Source: CAD feature listing. Evaluate the final solid. Frame: model axes, mm. Round coordinates to 2 decimals unless told otherwise and drop trailing zeros. Order: outer loops, then holes, each group sorted by start corner. A loop starts at its lowest first (then second) coordinate and runs counter-clockwise, first axis right, second up. Notation, with made-up numbers: (-37.5, 63.5) -> (5.5, 63.5) arc R26 cw to (5.5, 88.5) -> close; hole circle Ø2 at (-39.75, 89). An arc over 180 degrees is marked (long way). Write item = value, one per line. Start each with the question number.
(1) Draft query along Y for faces 1 (the face through (0, 34.29, 6)), 2 (the face through (31.75, -17, 6)), 3 (the face through (1.33, 0.35, 6.26)). Return one class per face: released by +Y, released by -Y, zero draft, split by the parting line, or undercut.
(2) Cut plane C-C on z = 4. Give the number of separate pieces and of enclosed holes in the cut face, then the cut area to 3 significant figures.
(3) Contact query for a flat-ended pin moving along its axis: pin 1 Ø7.5 at (x, y) = (-9.26, 0) entering from -Z. Output: stop coordinate, or through.
(4) Cut plane B-B on x = 5.5. Return the cut outline in (y, z), then the cut area to 3 significant figures.
(5) Ray query, line 1 (Y direction, x = -5, z = 9.75); line 2 (Y direction, x = 13.5, z = 9.5). Return the intervals inside material, ascending.
(6) Cut plane A-A on y = 0. Return the cut outline in (x, z).
from build123d import *

# Parameters (mm, degrees)
SKETCH1_W           = 63.5
SKETCH1_H           = 134.62
SKETCH1_R           = 6.35
SKETCH1_R_2         = 7.9375
BOSS_EXTRUDE1_DEPTH = 12.7
SKETCH2_W           = 63.5
SKETCH2_H           = 33.02
CUT_EXTRUDE1_DEPTH  = 76.498268854


with BuildPart() as part:
    # Sketch1 → Boss-Extrude1 (new body)
    with BuildSketch(Plane.XY):
        Rectangle(SKETCH1_W, SKETCH1_H)
        with Locations((-9.26084, 0)):
            Circle(SKETCH1_R, mode=Mode.SUBTRACT)
        with Locations((9.26084, 0)):
            Circle(SKETCH1_R_2, mode=Mode.SUBTRACT)
    extrude(amount=BOSS_EXTRUDE1_DEPTH)

    # Sketch2 → Cut-Extrude1 (cut, through all)
    with BuildSketch(Plane.XY.offset(12.7)):
        with Locations((0, 50.8)):
            Rectangle(SKETCH2_W, SKETCH2_H)
    extrude(amount=-CUT_EXTRUDE1_DEPTH, mode=Mode.SUBTRACT)


solid = part.part
Evaluation:
q1.face_1 = released by +Y
q1.face_2 = zero draft
q1.face_3 = undercut
q2.separate_pieces = 1
q2.enclosed_holes = 2
q2.area = 6,130 mm^2
q3.pin_1 = through
q4.outline = (-67.31, 0) -> (-6.99, 0) -> (-6.99, 12.7) -> (-67.31, 12.7) -> close; (6.99, 0) -> (34.29, 0) -> (34.29, 12.7) -> (6.99, 12.7) -> close
q4.area = 1,110 mm^2
q5.line_1 = -67.31 to -4.71, 4.71 to 34.29
q5.line_2 = -67.31 to -6.71, 6.71 to 34.29
q6.outline = (-31.75, 0) -> (-15.61, 0) -> (-15.61, 12.7) -> (-31.75, 12.7) -> close; (-2.91, 0) -> (1.32, 0) -> (1.32, 12.7) -> (-2.91, 12.7) -> close; (17.2, 0) -> (31.75, 0) -> (31.75, 12.7) -> (17.2, 12.7) -> close
